Solid Edge part; units mm, degrees
sketch "Sketch1" plane through (0, 0, 0) normal (0, -1, 0) x (1, 0, 0)
  line L0 (31.4924, 35.0939) -> (106.4924, 35.0939)
  line L1 (106.4924, 35.0939) -> (106.4924, 9.0939)
  line L2 (106.4924, 9.0939) -> (31.4924, 9.0939)
  line L3 (31.4924, 9.0939) -> (31.4924, 35.0939)
  dimension "D1" = 31.4924
  dimension "D2" = 106.4924
extrude "Protrusion1" add sketch "Sketch1" against normal blind 40
sketch "Sketch2" plane through (64.4924, 0, 22.0939) normal (0, -1, 0) x (1, 0, 0)
  line L0 (-26.5616, 2.8803) -> (-16.5, 3.7605)
  line L1 (-16.5, 3.7605) -> (-16.5, 11.0605)
  line L2 (-16.5, 11.0605) -> (26.14, 11.0605)
  line L3 (26.14, -11) -> (26.14, 11.0605)
  line L4 (-16.5, -11) -> (26.14, -11)
  line L5 (-16.5, -11) -> (-16.5, -3.7)
  line L6 (-16.5, -3.7) -> (-26.5616, -2.8197)
  line L7 (-26.5616, -2.8197) -> (-26.5616, 2.8803)
extrude "ExtrudedCutout_4" cut sketch "Sketch2" against normal blind 37
sketch "Sketch3" plane through (31.4924, 20, 22.0939) normal (-1, 0, 0) x (0, -1, 0)
  line L0 (-17, -4) -> (-17, 4)
  line L1 (-17, 4) -> (-12, 4)
  line L2 (-12, 4) -> (-12, -4)
  line L3 (-12, -4) -> (-17, -4)
  dimension "D1" = 17
  dimension "D2" = 17
  dimension "D3" = 12
extrude "Cutout1" cut sketch "Sketch3" against normal up to next
sketch "Sketch4" plane through (64.4924, 0, 22.0939) normal (0, -1, 0) x (1, 0, 0)
  line L0 (-16.5, 10.0605) -> (-25.5, 10.0605)
  line L1 (-25.5, 10.0605) -> (-25.5, -9.9395)
  line L2 (-25.5, -9.9395) -> (-16.5, -9.9395)
  line L3 (-16.5, -9.9395) -> (-16.5, 10.0605)
  line L4 (26.14, 10.0605) -> (35.14, 10.0605)
  line L5 (35.14, 10.0605) -> (35.14, -9.9395)
  line L6 (35.14, -9.9395) -> (26.14, -9.9395)
  line L7 (26.14, -9.9395) -> (26.14, 10.0605)
  dimension "D1" = 35.14
  dimension "D2" = 16.5
  dimension "D3" = 25.5
  dimension "D4" = 26.14
extrude "ExtrudedCutout_6" cut sketch "Sketch4" against normal blind 10
sketch "Sketch5" plane through (91.2324, 10, 21.645) normal (0, -1, 0) x (1, 0, 0)
  circle A0 centre (6.65, 5.5095) radius 2.25
  circle A1 centre (-50.49, 5.5095) radius 2.25
  circle A2 centre (-50.49, -4.4905) radius 2.25
  circle A3 centre (6.65, -4.4905) radius 2.25
  dimension "D1" = 50.49
  dimension "D2" = 6.65
  dimension "D3" = 50.49
extrude "ExtrudedCutout_7" cut sketch "Sketch5" against normal blind 5
sketch "Sketch6" plane through (64.4924, 0, 22.0939) normal (0, -1, 0) x (1, 0, 0)
  circle A0 centre (33.39, 5.0605) radius 2.25
  circle A1 centre (33.39, -4.9395) radius 2.25
  circle A2 centre (-23.75, 5.0605) radius 2.25
  circle A3 centre (-23.75, -4.9395) radius 2.25
extrude "Cutout2" cut sketch "Sketch6" against normal up to next
sketch "Sketch7" plane through (68.9924, 0, 22.0939) normal (0, -1, 0) x (1, 0, 0)
  line L0 (-31.0616, 11.0605) -> (32.14, 11.0605)
  line L1 (32.14, 11.0605) -> (32.14, -11)
  line L2 (32.14, -11) -> (-31.0616, -11)
  line L3 (-31.0616, -11) -> (-31.0616, 11.0605)
  line L4 (-37.5, 13) -> (-37.5, -13)
  line L5 (-37.5, -13) -> (37.5, -13)
  line L6 (37.5, -13) -> (37.5, 13)
  line L7 (37.5, 13) -> (-37.5, 13)
extrude "ExtrudedProtrusion_4" add sketch "Sketch7" along normal blind 15
sketch "Sketch8" plane through (68.9924, -15, 22.0939) normal (0, -1, 0) x (1, 0, 0)
  circle A0 centre (-12.76, 0) radius 22.5
extrude "ExtrudedCutout_9" cut sketch "Sketch8" against normal blind 15
Read the model definition and answer for the solid it produces. Units are mm, in the model's axes. A direction names the side the tool comes from. Coordinates: 2 decimals unless noted, no trailing zeros. Write each loop counter-clockwise with the first axis right and the second up, starting at its lowest first coordinate (ties: lowest second). Pieces come first, ordered by that corner, then holes. Notation, with made-up numbers: (48.5, -4) -> (63.5, -4) arc R19 cw to (63.5, 28) -> close; hole circle Ø5 at (-21, 26.5). An arc over 180 degrees is marked (long way). Write item = value, one per line.
(1) Straight lines are drawn through the part: L1, parallel to Z at x = 65.5, y = 9; L2, parallel to X at y = 11, z = 23.5; L3, parallel to Y at x = 49, z = 22.5. For each, find the intervals that lie inside material, in ascending order. Write a range as from..to.
From the geometry:
L1 = 9.09..11.09, 33.15..35.09
L2 = 31.49..37.93, 90.63..106.49
L3 = 37..40
(2) Given pin 1 Ø6.5 at (x, z) = (54, 19.5) entering from -Y; pin 2 Ø5.5 at (x, z) = (42.5, 28) entering from -Y; pin 3 Ø8 at (x, z) = (42.5, 20) entering from -Y, each flat-ended and moving along its own axis, determine where each tip first touches the part or whether it passes through.
From the geometry:
pin_1 = 37
pin_2 = 10
pin_3 = 0
(3) Section A-A on y = -5 is taken. Write down the section's boundary in (x, z), plus the area to 3 significant figures.
From the geometry:
outline = (31.49, 9.09) -> (37.87, 9.09) arc R22.5 cw to (37.87, 35.09) -> (31.49, 35.09) -> close; (74.6, 9.09) -> (106.49, 9.09) -> (106.49, 35.09) -> (74.6, 35.09) arc R22.5 cw to (75.83, 33.15) -> (101.13, 33.15) -> (101.13, 11.09) -> (75.86, 11.09) arc R22.5 cw to start
area = 334 mm2
(4) Which of the six approach directions +Z, -Z, +X, -X, +Y, -Y give full straight-line access (tool end or side, diameter ignored) to faces 1 (the face through (41, 15, 17)), 2 (the face through (70, 18, 9.094))?
From the geometry:
face_1 = -Y
face_2 = -Z, +X, -X, +Y, -Y
(5) Section D-D on z = 20.75 is taken. Write down the section's boundary in (x, y).
From the geometry:
outline = (31.49, -15) -> (33.77, -15) -> (33.77, 0) -> (37.93, 0) -> (37.93, 32) -> (31.49, 32) -> close; (31.49, 37) -> (90.63, 37) -> (90.63, 10) -> (99.63, 10) -> (99.63, 0) -> (101.13, 0) -> (101.13, -15) -> (106.49, -15) -> (106.49, 40) -> (31.49, 40) -> close
(6) Section C-C on x = 84.5 is taken. Write down the section's boundary in (y, z), plus the area to 3 significant figures.
From the geometry:
outline = (-15, 9.09) -> (40, 9.09) -> (40, 35.09) -> (-15, 35.09) -> (-15, 33.15) -> (37, 33.15) -> (37, 11.09) -> (-15, 11.09) -> close
area = 283 mm2
(7) Section B-B on y = 28 is taken. Write down the section's boundary in (x, z), plus the area to 3 significant figures.
From the geometry:
outline = (31.49, 9.09) -> (106.49, 9.09) -> (106.49, 35.09) -> (31.49, 35.09) -> close; hole (37.93, 19.27) -> (47.99, 18.39) -> (47.99, 11.09) -> (90.63, 11.09) -> (90.63, 33.15) -> (47.99, 33.15) -> (47.99, 25.85) -> (37.93, 24.97) -> close
area = 943 mm2
(8) For a pull along Y with two mould halves and no side action, classify faces 3 (the face through (40, 34, 18.094)), 4 (the face through (106.492, 12, 22)), 5 (the face through (33, -15, 22)) as +Y half, -Y half, draft (parallel to the pull), parting line (faces both ways), or undercut.
From the geometry:
face_3 = undercut
face_4 = draft
face_5 = -Y half
